Read the model definition and answer for the solid it produces. Units are mm, in the model's axes. Face numbers are marked on the shaded views. A direction names the side the tool comes from. Coordinates: 2 decimals unless noted, no trailing zeros. Order: outer loops, then holes, each group sorted by start corner. A loop starts at its lowest first (then second) coordinate and runs counter-clockwise, first axis right, second up. Notation, with made-up numbers: (-23.75, 65) -> (29.25, 65) arc R18 ccw to (29.25, 76) -> close; hole circle Ø6 at (-2, 76.5). An arc over 180 degrees is marked (long way). Answer in a Markdown table with one row per item.
from build123d import *

# Parameters (mm, degrees)
BOSS_EXTRUDE1_DEPTH             = 3.032500031
BOSS_EXTRUDE2_REACH             = 21.994
BOSS_EXTRUDE2_DIRECTION_2_REACH = 21.994
CUT_EXTRUDE1_DEPTH              = 30.326387225


with BuildPart() as part:
    # Sketch1 → Boss-Extrude1 (new, symmetric)
    with BuildSketch(Plane.XY):
        Polygon((-3.9525, -18.875), (-5.8575, -18.875), (-5.8575, 18.875), (-3.9525, 18.875), (-2.6825, 17.605), (-2.6825, -17.605), align=None)
    extrude(amount=BOSS_EXTRUDE1_DEPTH, both=True)

    # Boss-Extrude2: up to this face of the body (flat: up to its plane)
    boss_extrude2_end = Plane(part.part.faces().sort_by_distance((-4.285879831, 0, 3.032500031))[0])
    # Sketch1<3> → Boss-Extrude2 (add, up to the picked face)
    with BuildSketch(Plane.XY, mode=Mode.PRIVATE) as boss_extrude2_sk1:
        Polygon((-2.6825, 13.16), (-2.6825, 9.7), (4.5875, 9.7), (5.8575, 10.97), (5.8575, 13.16), align=None)
    boss_extrude2_tool1 = split(extrude(boss_extrude2_sk1.sketch, amount=BOSS_EXTRUDE2_REACH, mode=Mode.PRIVATE), bisect_by=boss_extrude2_end, keep=Keep.BOTH, mode=Mode.PRIVATE)
    # Sketch1<3> → Boss-Extrude2 (add, up to the picked face)
    with BuildSketch(Plane.XY, mode=Mode.PRIVATE) as boss_extrude2_sk2:
        Polygon((-2.6825, 15.7), (-2.6825, 14.43), (5.8575, 14.43), (5.8575, 14.938), (4.4605, 16.335), (3.9525, 16.335), (3.3175, 15.7), align=None)
    boss_extrude2_tool2 = split(extrude(boss_extrude2_sk2.sketch, amount=BOSS_EXTRUDE2_REACH, mode=Mode.PRIVATE), bisect_by=boss_extrude2_end, keep=Keep.BOTH, mode=Mode.PRIVATE)
    add(boss_extrude2_tool1.solids().sort_by(Axis((1.479569, 11.466663, 0), (0, 0, 1)))[0])
    add(boss_extrude2_tool2.solids().sort_by(Axis((1.652648, 15.112693, 0), (0, 0, 1)))[0])

    # Boss-Extrude2 direction 2: up to this face of the body (flat: up to its plane)
    boss_extrude2_direction_2_end = Plane(part.part.faces().sort_by_distance((-4.285879831, 0, -3.032500031))[0])
    # Sketch1<3> → Boss-Extrude2 direction 2 (add, up to the picked face)
    with BuildSketch(Plane.XY, mode=Mode.PRIVATE) as boss_extrude2_direction_2_sk1:
        Polygon((-2.6825, 13.16), (-2.6825, 9.7), (4.5875, 9.7), (5.8575, 10.97), (5.8575, 13.16), align=None)
    boss_extrude2_direction_2_tool1 = split(extrude(boss_extrude2_direction_2_sk1.sketch, amount=-BOSS_EXTRUDE2_DIRECTION_2_REACH, mode=Mode.PRIVATE), bisect_by=boss_extrude2_direction_2_end, keep=Keep.BOTH, mode=Mode.PRIVATE)
    # Sketch1<3> → Boss-Extrude2 direction 2 (add, up to the picked face)
    with BuildSketch(Plane.XY, mode=Mode.PRIVATE) as boss_extrude2_direction_2_sk2:
        Polygon((-2.6825, 15.7), (-2.6825, 14.43), (5.8575, 14.43), (5.8575, 14.938), (4.4605, 16.335), (3.9525, 16.335), (3.3175, 15.7), align=None)
    boss_extrude2_direction_2_tool2 = split(extrude(boss_extrude2_direction_2_sk2.sketch, amount=-BOSS_EXTRUDE2_DIRECTION_2_REACH, mode=Mode.PRIVATE), bisect_by=boss_extrude2_direction_2_end, keep=Keep.BOTH, mode=Mode.PRIVATE)
    add(boss_extrude2_direction_2_tool1.solids().sort_by(Axis((1.479569, 11.466663, 0), (0, 0, -1)))[0])
    add(boss_extrude2_direction_2_tool2.solids().sort_by(Axis((1.652648, 15.112693, 0), (0, 0, -1)))[0])

    # Sketch2 → Cut-Extrude1 (cut, through all)
    with BuildSketch(Plane.XZ.offset(-9.7)):
        Polygon((3.3175, 3.032500031), (5.8575, 1.762500031), (5.8575, 3.032500031), align=None)
    extrude(amount=-CUT_EXTRUDE1_DEPTH, mode=Mode.SUBTRACT)

    # Mirror2: part across plane


with BuildPart() as part_1:
    add(part.part)
    add(part.part.mirror(Plane.ZX))


solid = part_1.part
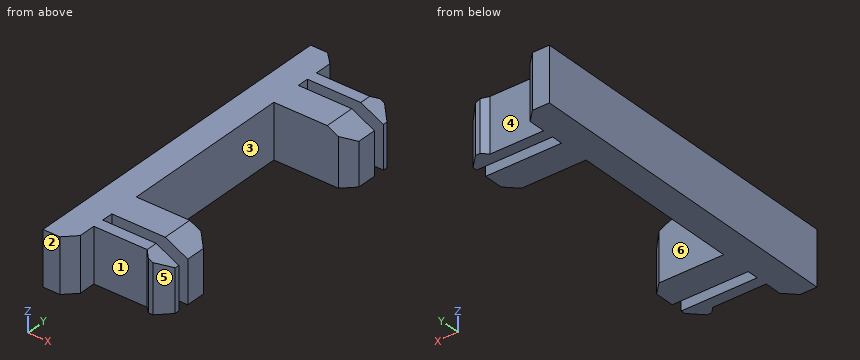
Q1. For a pull along Y with two mould halves and no side action, classify the marked faces 4, 5 and 6 as pulls with the +Y half, pulls with the -Y half, needs draft (parallel to the pull), parting line crosses it, or undercut.
Outcome:
| item | result |
|---|---|
| face 4 | pulls with the +Y half |
| face 5 | pulls with the -Y half |
| face 6 | undercut |
Q2. Consider line 1 (Y direction, x = 4, z = -1.5) (3 decimals); line 2 (Y direction, x = 2, z = -2.5); line 3 (X direction, y = -9, z = 2.5). Determine where each line is inside the solid, lowest interval first.
Outcome:
| item | result |
|---|---|
| line 1 | -16.335 to -14.43, -13.16 to -9.7, 9.7 to 13.16, 14.43 to 16.335 |
| line 2 | -15.7 to -14.43, -13.16 to -9.7, 9.7 to 13.16, 14.43 to 15.7 |
| line 3 | -5.86 to -2.68 |
Q3. The part is cut by section A-A (x = 2). Write down the section's boundary in (y, z).
Outcome:
| item | result |
|---|---|
| outline | (-15.7, -3.03) -> (-14.43, -3.03) -> (-14.43, 3.03) -> (-15.7, 3.03) -> close; (-13.16, -3.03) -> (-9.7, -3.03) -> (-9.7, 3.03) -> (-13.16, 3.03) -> close; (9.7, -3.03) -> (13.16, -3.03) -> (13.16, 3.03) -> (9.7, 3.03) -> close; (14.43, -3.03) -> (15.7, -3.03) -> (15.7, 3.03) -> (14.43, 3.03) -> close |
Q4. The part is cut by section C-C (y = -9). Write down the section's boundary in (x, z), then the cut area to 3 significant figures.
Outcome:
| item | result |
|---|---|
| outline | (-5.86, -3.03) -> (-2.68, -3.03) -> (-2.68, 3.03) -> (-5.86, 3.03) -> close |
| area | 19.3 mm² |
Q5. For the marked faces 1, 2 and 3, determine the directions among +Z, -Z, +X, -X, +Y, -Y from which every point of the face is accessible in a straight line to the end or side of a thin tool.
Outcome:
| item | result |
|---|---|
| face 1 | +Z, -Z, -Y |
| face 2 | +Z, -Z, +X, -X, -Y |
| face 3 | +Z, -Z, +X |
Q6. Given pin 1 (2 mm diameter, centred on y = -17, z = -1, fed in from +X); pin 2 (0.6 mm diameter, centred on y = -14, z = 0.5, fed in from +X); pin 3 (3 mm diameter, centred on x = 2, z = -0.5, fed in from -Y); pin 4 (1 mm diameter, centred on x = 3, y = -14, fed in from -Z), each flat-ended and moving along its own axis, determine where each tip first touches the part or whether it passes through.
Outcome:
| item | result |
|---|---|
| pin 1 | x = 4.8 |
| pin 2 | x = -2.68 |
| pin 3 | y = -15.88 |
| pin 4 | z = -3.03 |
